```python
from build123d import *

# Parameters (mm, degrees)
CROQUIS1_R              = 64
CROQUIS1_R_2            = 61
SALIENTE_EXTRUIR1_DEPTH = 3.9
SALIENTE_EXTRUIR2_START = 2
CROQUIS2_R              = 64
CROQUIS2_R_2            = 62.5
SALIENTE_EXTRUIR2_DEPTH = 2
SALIENTE_EXTRUIR3_START = 0.5
CROQUIS3_R              = 64
CROQUIS3_R_2            = 61
SALIENTE_EXTRUIR3_DEPTH = 0.5


with BuildPart() as part:
    # Croquis1 → Saliente-Extruir1 (new body)
    with BuildSketch(Plane(origin=(0, 0, 0), x_dir=(1, 0, 0), z_dir=(0, 1, 0))):
        with Locations(Location((0, 0, 0), (0, 0, 270))):
            Circle(CROQUIS1_R)
        with Locations(Location((0, 0, 0), (0, 0, 270))):
            Circle(CROQUIS1_R_2, mode=Mode.SUBTRACT)
    extrude(amount=SALIENTE_EXTRUIR1_DEPTH)

    # Croquis2 → Saliente-Extruir2 (add)
    with BuildSketch(Plane.XZ.offset(SALIENTE_EXTRUIR2_START)):
        with Locations(Location((0, 0, 0), (0, 0, 270))):
            Circle(CROQUIS2_R)
        with Locations(Location((0, 0, 0), (0, 0, 270))):
            Circle(CROQUIS2_R_2, mode=Mode.SUBTRACT)
    extrude(amount=-SALIENTE_EXTRUIR2_DEPTH)

    # Croquis3 → Saliente-Extruir3 (add)
    with BuildSketch(Plane.XZ.offset(2).offset(SALIENTE_EXTRUIR3_START)):
        with Locations(Location((0, 0, 0), (0, 0, 270))):
            Circle(CROQUIS3_R)
        with Locations(Location((0, 0, 0), (0, 0, 90))):
            Circle(CROQUIS3_R_2, mode=Mode.SUBTRACT)
    extrude(amount=-SALIENTE_EXTRUIR3_DEPTH)


solid = part.part
```
Read the model definition and answer for the solid it produces. Units are mm, in the model's axes. A direction names the side the tool comes from. Coordinates: 2 decimals unless noted, no trailing zeros. Order: outer loops, then holes, each group sorted by start corner. A loop starts at its lowest first (then second) coordinate and runs counter-clockwise, first axis right, second up. Notation, with made-up numbers: (24, -22) - (47, -22) arc R32 ccw to (47, 16) - close; hole circle Ø3 at (-25, -17). An arc over 180 degrees is marked (long way). Answer as a JSON object with one key per item and string values. Group by question number.
Item 1: A tool of negligible diameter and unlimited length cuts with its end or side. For faces 1 (the face through (59.55, -2.25, -13.22)), 2 (the face through (-60, -2, -14)), from which of +Z, -Z, +X, -X, +Y, -Y can it reach the whole face along a straight path? Write none if from no direction.
Item 2: Section C-C (y = 2.25) is taken. Give the vertices of the cut face in (x, z).
Item 3: Flat-ended cylindrical pins translate along their axes: P1, Ø2, axis at x = -7.5, y = -0.5, coming from the -Z side; P2, Ø1.5, axis at y = -1.5, z = 10.5, coming from the +X side; P3, Ø3, axis at x = -37.5, y = 0.5, coming from the +Z side (3 decimals). Find the tip coordinate at first contact, or state that the pin passes through.
Item 4: Section B-B (z = 0) is taken. Give the vertices of the cut face in (x, y), plus the area to 3 significant figures.
Item 5: Section A-A (x = 0) is taken. Give the vertices of the cut face in (y, z).
Item 6: Consider probe 1 along X at (y, z) = (2.65, 0); probe 2 along X at (y, z) = (-1.1, 0); probe 3 along Z at (x, y) = (43.5, 1.25). Determine where each line is inside the solid, lowest interval first. Write a range as from..to.
Item 7: The mould has two halves that part along Y. Classify faces 3 (the face through (-23, -2.5, -57)), 4 (the face through (2.75, -1.01, 62.44)), 5 (the face through (-59.55, 1.92, -13.22)): +Y half, -Y half, draft (parallel to the pull), parting line (faces both ways), or undercut.
Results are:
{
 "1": {"face 1": "+Y, -Y", "face 2": "none"},
 "2": {"outline": "circle Ø128 at (0, 0); hole circle Ø122 at (0, 0)"},
 "3": {"P1": "stops at z = -63.67", "P2": "stops at x = 63.25", "P3": "stops at z = 52.915"},
 "4": {"outline": "(-64, -2.5) - (-61, -2.5) - (-61, -2) - (-62.5, -2) - (-62.5, 0) - (-61, 0) - (-61, 3.9) - (-64, 3.9) - close; (61, -2.5) - (64, -2.5) - (64, 3.9) - (61, 3.9) - (61, 0) - (62.5, 0) - (62.5, -2) - (61, -2) - close", "area": "32.4 mm^2"},
 "5": {"outline": "(-2.5, -64) - (3.9, -64) - (3.9, -61) - (0, -61) - (0, -62.5) - (-2, -62.5) - (-2, -61) - (-2.5, -61) - close; (-2.5, 61) - (-2, 61) - (-2, 62.5) - (0, 62.5) - (0, 61) - (3.9, 61) - (3.9, 64) - (-2.5, 64) - close"},
 "6": {"probe 1": "x = -64..-61, 61..64", "probe 2": "x = -64..-62.5, 62.5..64", "probe 3": "z = -46.94..-42.76, 42.76..46.94"},
 "7": {"face 3": "-Y half", "face 4": "undercut", "face 5": "draft"}
}
